Part model, mm, in its own coordinate system. A direction names the side the tool comes from. Round coordinates to 2 decimals unless told otherwise and drop trailing zeros. Order: outer loops, then holes, each group sorted by start corner. A loop starts at its lowest first (then second) coordinate and runs counter-clockwise, first axis right, second up. Notation, with made-up numbers: (66.25, -27) - (114.25, -27) arc R11 cw to (114.25, -9) - close; hole circle Ø6 at (77.5, 18.5). An arc over 180 degrees is marked (long way). Answer as a JSON object with one key per item and string values.
```python
from build123d import *

# Parameters (mm, degrees)
SKETCH1_R           = 1.65
SKETCH1_R_2         = 1.6
SKETCH1_R_3         = 12.5
SKETCH1_R_4         = 2.2
SKETCH1_R_5         = 4
BOSS_EXTRUDE1_DEPTH = 7.5


with BuildPart() as part:
    # Sketch1 → Boss-Extrude1 (new body)
    with BuildSketch(Plane(origin=(0, 3.75, 0), x_dir=(1, 0, 0), z_dir=(0, 1, 0))):
        with BuildLine():
            Line((34.035533906, 17.464466094), (31.964466094, 19.535533906))
            ThreePointArc((31.964466094, 19.535533906), (30.34234935, 20.619397663), (28.428932188, 21))
            Line((28.428932188, 21), (15.071067812, 21))
            ThreePointArc((15.071067812, 21), (13.15765065, 21.380602337), (11.535533906, 22.464466094))
            Line((11.535533906, 22.464466094), (9.464466094, 24.535533906))
            ThreePointArc((9.464466094, 24.535533906), (8.380602337, 26.15765065), (8, 28.071067812))
            Line((8, 28.071067812), (8, 68))
            ThreePointArc((8, 68), (6.535533906, 71.535533906), (3, 73))
            Line((3, 73), (-22.5, 73))
            ThreePointArc((-22.5, 73), (-26.035533906, 71.535533906), (-27.5, 68))
            Line((-27.5, 68), (-27.5, -68))
            ThreePointArc((-27.5, -68), (-26.035533906, -71.535533906), (-22.5, -73))
            Line((-22.5, -73), (3, -73))
            ThreePointArc((3, -73), (6.535533906, -71.535533906), (8, -68))
            Line((8, -68), (8, -28.071067812))
            ThreePointArc((8, -28.071067812), (8.380602337, -26.15765065), (9.464466094, -24.535533906))
            Line((9.464466094, -24.535533906), (11.535533906, -22.464466094))
            ThreePointArc((11.535533906, -22.464466094), (13.15765065, -21.380602337), (15.071067812, -21))
            Line((15.071067812, -21), (28.428932188, -21))
            ThreePointArc((28.428932188, -21), (30.34234935, -20.619397663), (31.964466094, -19.535533906))
            Line((31.964466094, -19.535533906), (34.035533906, -17.464466094))
            ThreePointArc((34.035533906, -17.464466094), (35.119397663, -15.84234935), (35.5, -13.928932188))
            Line((35.5, -13.928932188), (35.5, 13.928932188))
            ThreePointArc((35.5, 13.928932188), (35.119397663, 15.84234935), (34.035533906, 17.464466094))
        make_face()
        with Locations((0, -68)):
            Circle(SKETCH1_R, mode=Mode.SUBTRACT)
        with Locations((0, -52)):
            Circle(SKETCH1_R, mode=Mode.SUBTRACT)
        with Locations((0, 68)):
            Circle(SKETCH1_R, mode=Mode.SUBTRACT)
        with Locations((0, 52)):
            Circle(SKETCH1_R, mode=Mode.SUBTRACT)
        with Locations((29.5, 15.5)):
            Circle(SKETCH1_R_2, mode=Mode.SUBTRACT)
        with Locations((-1.5, 15.5)):
            Circle(SKETCH1_R_2, mode=Mode.SUBTRACT)
        with Locations((-1.5, -15.5)):
            Circle(SKETCH1_R_2, mode=Mode.SUBTRACT)
        with Locations((29.5, -15.5)):
            Circle(SKETCH1_R_2, mode=Mode.SUBTRACT)
        with Locations((14, 0)):
            Circle(SKETCH1_R_3, mode=Mode.SUBTRACT)
        with Locations((-17.5, 0)):
            Circle(SKETCH1_R_4, mode=Mode.SUBTRACT)
        with Locations((0, -60)):
            Circle(SKETCH1_R_5, mode=Mode.SUBTRACT)
        with Locations((0, 60)):
            Circle(SKETCH1_R_5, mode=Mode.SUBTRACT)
        with Locations((-17.5, 60)):
            Circle(SKETCH1_R_4, mode=Mode.SUBTRACT)
        with Locations((-17.5, -60)):
            Circle(SKETCH1_R_4, mode=Mode.SUBTRACT)
    extrude(amount=-BOSS_EXTRUDE1_DEPTH)


solid = part.part
```
Item 1: Cut at A-A (x = -17.5). Write the cut outline in (y, z).
Taken from the geometry:
{"outline": "(-3.75, -73) - (3.75, -73) - (3.75, -62.2) - (-3.75, -62.2) - close; (-3.75, -57.8) - (3.75, -57.8) - (3.75, -2.2) - (-3.75, -2.2) - close; (-3.75, 2.2) - (3.75, 2.2) - (3.75, 57.8) - (-3.75, 57.8) - close; (-3.75, 62.2) - (3.75, 62.2) - (3.75, 73) - (-3.75, 73) - close"}
Item 2: Tool access for faces 1 (the flat face through (8, 0, -48)), 2 (the flat face through (8, 0, 48)), 3 (the cylindrical face through (0.89, 0.05, 50.61)): list every direction of +Z, -Z, +X, -X, +Y, -Y with a clear straight run to the whole face (end or side of a thin tool).
Taken from the geometry:
{"face 1": "-Z, +X, +Y, -Y", "face 2": "+Z, +X, +Y, -Y", "face 3": "+Y, -Y"}
Item 3: Cut at B-B (z = -15.5). Write the cut outline in (x, y).
Taken from the geometry:
{"outline": "(-27.5, -3.75) - (-3.1, -3.75) - (-3.1, 3.75) - (-27.5, 3.75) - close; (0.1, -3.75) - (27.9, -3.75) - (27.9, 3.75) - (0.1, 3.75) - close; (31.1, -3.75) - (35.25, -3.75) - (35.25, 3.75) - (31.1, 3.75) - close"}
Item 4: Two-plate mould, pull along Z, no slides. Class faces 4 (the cylindrical face through (30.32, 0.05, 20.63)), 5 (the flat face through (-3, 3.75, -1)), 6 (the cylindrical face through (-15.468, 0.053, 0.843)): pulls with the +Z half, pulls with the -Z half, needs draft (parallel to the pull), parting line crosses it, or undercut.
Taken from the geometry:
{"face 4": "pulls with the +Z half", "face 5": "needs draft", "face 6": "undercut"}
Item 5: Probe L1, parallel to X at y = 1, z = 60; L2, parallel to Z at x = -17.5, y = -2; L3, parallel to X at y = -0.5, z = -68. List the from-to ranges inside material, lowest first. Write a range as from..to.
Taken from the geometry:
{"L1": "-27.5..-19.7, -15.3..-4, 4..8", "L2": "-73..-62.2, -57.8..-2.2, 2.2..57.8, 62.2..73", "L3": "-27.5..-1.65, 1.65..8"}
Item 6: Drop flat-ended pins along their axis: P1, Ø2, axis at x = 20, y = 1.5, coming from the -Z side; P2, Ø4, axis at x = 15.5, y = -0.5, coming from the -Z side; P3, Ø4, axis at x = 6.5, y = -3, coming from the +Z side. Give the stop position or say it passes through.
Taken from the geometry:
{"P1": "z = -21", "P2": "z = -21.25", "P3": "z = 72.77"}
Item 7: Cut at C-C (x = 18). Write the cut outline in (y, z), plus the area to 3 significant figures.
Taken from the geometry:
{"outline": "(-3.75, -21) - (3.75, -21) - (3.75, -11.84) - (-3.75, -11.84) - close; (-3.75, 11.84) - (3.75, 11.84) - (3.75, 21) - (-3.75, 21) - close", "area": "137 mm2"}
Item 8: Cut at D-D (y = 0.75). State how many separate pieces and enclosed holes the cut face has, plus the area to 3 significant figures.
Taken from the geometry:
{"separate pieces": "1", "enclosed holes": "14", "area": "5,610 mm2"}
